Geometry check sheet. Reference: drawing and pictorial views, mm from the part's lowest x, y, z. A direction names the side the tool comes from. Round coordinates to 2 decimals unless told otherwise and drop trailing zeros. Loops run counter-clockwise (first coordinate to the right, second up) from the corner with the lowest first, then second, coordinate; pieces in that order, holes last. Notation, with made-up numbers: (53, 34.5) - (109, 34.5) arc R17 ccw to (109, 52.5) - close; hole circle Ø9 at (50.25, 24.5). An arc over 180 degrees is marked (long way). Return JSON: item names as keys, results as strings.
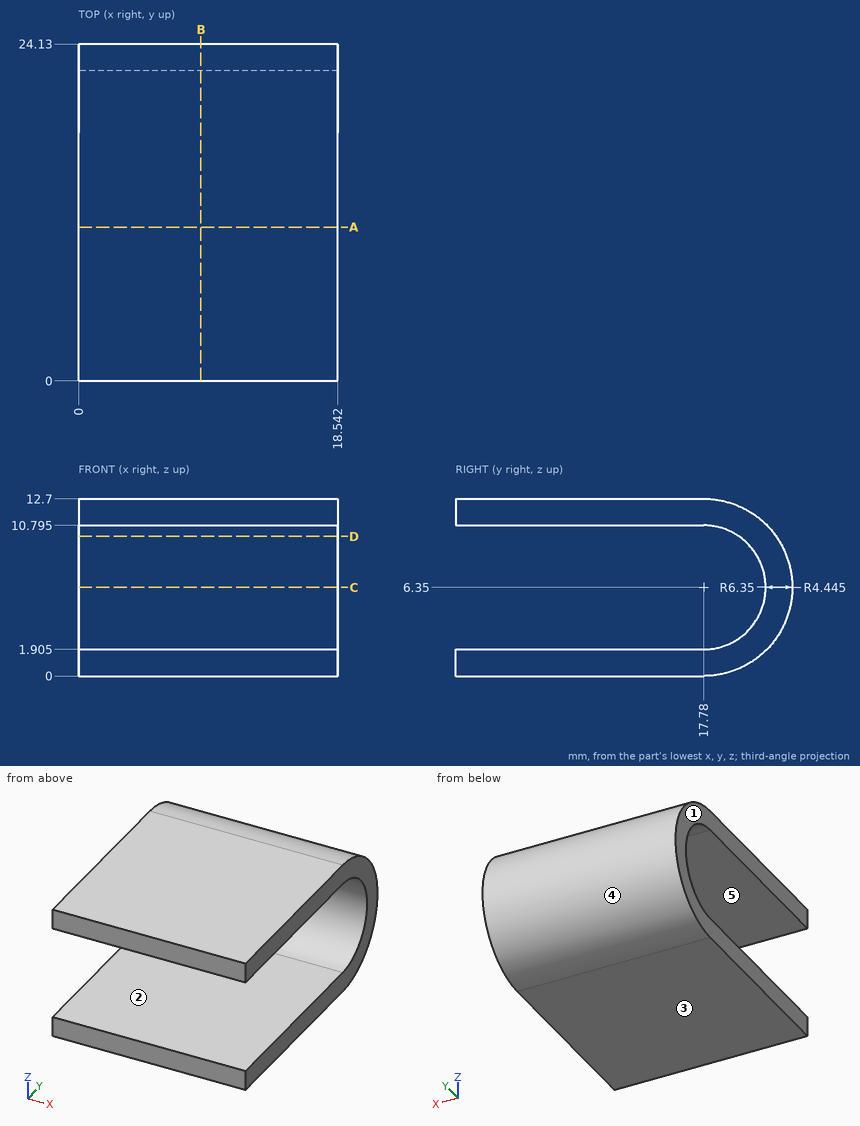
Q1. Tool access check on the marked faces 4 and 5. Record the directions out of +Z, -Z, +X, -X, +Y, -Y that give a thin tool (end or side, any length) a straight path to the whole face; none if there is none.
Answer key:
{"face 4": "+X, -X, +Y", "face 5": "+X, -X, -Y"}
Q2. Sectioned sample at C-C (z = 6.35). Enter the section's corners in (x, y) (3 decimals).
Answer key:
{"outline": "(0, 22.225) - (18.542, 22.225) - (18.542, 24.13) - (0, 24.13) - close"}
Q3. Sectioned sample at A-A (y = 11). Enter the section's corners in (x, z) (3 decimals), plus the area to 3 significant figures.
Answer key:
{"outline": "(0, 0) - (18.542, 0) - (18.542, 1.905) - (0, 1.905) - close; (0, 10.795) - (18.542, 10.795) - (18.542, 12.7) - (0, 12.7) - close", "area": "70.6 mm²"}
Q4. Sectioned sample at B-B (x = 8.75). Enter the section's corners in (y, z) (3 decimals).
Answer key:
{"outline": "(0, 0) - (17.78, 0) arc R6.35 ccw to (17.78, 12.7) - (0, 12.7) - (0, 10.795) - (17.78, 10.795) arc R4.445 cw to (17.78, 1.905) - (0, 1.905) - close"}
Q5. Sectioned sample at D-D (z = 10). Enter the section's corners in (x, y), plus the area to 3 significant figures.
Answer key:
{"outline": "(0, 20.32) - (18.54, 20.32) - (18.54, 22.98) - (0, 22.98) - close", "area": "49.3 mm²"}
Q6. Scan lines: probe 1 along Z at (x, y) = (6, 17.25) (3 decimals); probe 2 along Z at (x, y) = (3, 19); probe 3 along Y at (x, z) = (1.5, 8.5). Record each from-to range of solid material in increasing order. Write a range as [from, to].
Answer key:
{"probe 1": "z = [0, 1.905], [10.795, 12.7]", "probe 2": "z = [0.12, 2.08], [10.62, 12.58]", "probe 3": "y = [21.67, 23.75]"}
Q7. Draft check along Z on the marked faces 1, 2 and 3. Enter one of: released by +Z, released by -Z, zero draft, split by the parting line, or undercut.
Answer key:
{"face 1": "zero draft", "face 2": "undercut", "face 3": "released by -Z"}
